from build123d import *

# Parameters (mm, degrees)
SKETCH_1_R                = 39.75
EXTRUDE_1_DEPTH           = 10
SKETCH_7_R                = 2.65
CUT_EXTRUDE_5_DEPTH       = 8
PATTERN_CIRCULAR_1_COUNT  = 2
PATTERN_CIRCULAR_1_ANGLE  = 25
F_1_THE_OTHER_WAY_COUNT   = 2
F_1_THE_OTHER_WAY_ANGLE   = 25
MIRROR_1_COPY_1_SKETCH_R  = 2.65
MIRROR_1_COPY_1_DEPTH     = 8
MIRROR_1_COPY_2_SKETCH_R  = 2.65
MIRROR_1_COPY_2_DEPTH     = 8
SKETCH_9_R                = 2.65
CUT_EXTRUDE_7_DEPTH       = 8
PATTERN_CIRCULAR_2_COUNT  = 2
CUT_EXTRUDE_START         = -10
CUT_EXTRUDE_8_DEPTH       = 10
CUT_EXTRUDE_13_DEPTH      = 4
SKETCH_12_R               = 25
EXTRUDE_2_DEPTH           = 10
SKETCH_16_R               = 21.4
CUT_EXTRUDE_14_DEPTH      = 6
CUT_EXTRUDE_10_DEPTH      = 58.09750448
CUT_EXTRUDE_10_DEPTH_BACK = 58.09750448
SKETCH_13_R               = 2.25
SKETCH_13_R_2             = 13.5
SKETCH_17_R               = 4.25
CUT_EXTRUDE_15_DEPTH      = 8
FILLET_1_R                = 2.5


# Read off the part's stored shape, not the designer's step: Вырез-Вытянуть8
with BuildPart() as part:
    # Эскиз1 → Бобышка-Вытянуть1 (new body)
    with BuildSketch(Plane.XY):
        Circle(SKETCH_1_R)
    extrude(amount=EXTRUDE_1_DEPTH)

    # Эскиз7 → Вырез-Вытянуть5 (cut)
    with BuildSketch(Plane(origin=(0, 39.75, 0), x_dir=(0, 0, -1), z_dir=(0, 1, 0))):
        with Locations(Location((-5, 0, 0), (0, 0, 90))):
            Circle(SKETCH_7_R)
    cut_extrude_5 = extrude(amount=-CUT_EXTRUDE_5_DEPTH, mode=Mode.SUBTRACT)

    # Круговой массив1: Вырез-Вытянуть5 ×2 about axis
    pattern_circular_1_axis = Axis((0, 0, 10), (0, 0, -1))
    for i in range(1, PATTERN_CIRCULAR_1_COUNT):
        add(cut_extrude_5.rotate(pattern_circular_1_axis, i * PATTERN_CIRCULAR_1_ANGLE / (PATTERN_CIRCULAR_1_COUNT - 1)), mode=Mode.SUBTRACT)

    # 1 the other way: Вырез-Вытянуть5 ×2 about axis
    f_1_the_other_way_axis = Axis((0, 0, 10), (0, 0, 1))
    for i in range(1, F_1_THE_OTHER_WAY_COUNT):
        add(cut_extrude_5.rotate(f_1_the_other_way_axis, i * F_1_THE_OTHER_WAY_ANGLE / (F_1_THE_OTHER_WAY_COUNT - 1)), mode=Mode.SUBTRACT)

    # Зеркальное отражение1: Вырез-Вытянуть5 across plane
    add(cut_extrude_5.mirror(Plane.ZX), mode=Mode.SUBTRACT)

    # Зеркальное отражение1 copy 1 sketch → Зеркальное отражение1 copy 1 (cut)
    with BuildSketch(Plane(origin=(16.799075904, -36.025734535, 0), x_dir=(0, 0, -1), z_dir=(0.4226182617407035, -0.906307787036648, 0))):
        with Locations((-5, 0)):
            Circle(MIRROR_1_COPY_1_SKETCH_R)
    extrude(amount=-MIRROR_1_COPY_1_DEPTH, mode=Mode.SUBTRACT)

    # Зеркальное отражение1 copy 2 sketch → Зеркальное отражение1 copy 2 (cut)
    with BuildSketch(Plane(origin=(-16.799075904, -36.025734535, 0), x_dir=(0, 0, -1), z_dir=(-0.42261826174069717, -0.9063077870366509, 0))):
        with Locations((-5, 0)):
            Circle(MIRROR_1_COPY_2_SKETCH_R)
    extrude(amount=-MIRROR_1_COPY_2_DEPTH, mode=Mode.SUBTRACT)

    # Эскиз9 → Вырез-Вытянуть7 (cut)
    with BuildSketch(Plane.ZY.offset(39.75)):
        with Locations((5, 0)):
            Circle(SKETCH_9_R)
    cut_extrude_7 = extrude(amount=-CUT_EXTRUDE_7_DEPTH, mode=Mode.SUBTRACT)

    # Круговой массив2: Вырез-Вытянуть7 ×2 about axis
    pattern_circular_2_axis = Axis((0, 0, 10), (0, 0, -1))
    for i in range(1, PATTERN_CIRCULAR_2_COUNT):
        add(cut_extrude_7.rotate(pattern_circular_2_axis, i * 360 / PATTERN_CIRCULAR_2_COUNT), mode=Mode.SUBTRACT)

    # Вырез-Вытянуть8 outline → Вырез-Вытянуть8 (cut)
    with BuildSketch(Plane(origin=(0, 0, 0), x_dir=(-1, 0, 0), z_dir=(0, 0, -1)).offset(CUT_EXTRUDE_START)):
        with BuildLine():
            Line((36.811173575, 15), (26.811173575, 15))
            Line((26.811173575, 15), (26.811173575, -15))
            Line((26.811173575, -15), (36.811173575, -15))
            ThreePointArc((36.811173575, -15), (39.75, 0), (36.811173575, 15))
        make_face()
    extrude(amount=CUT_EXTRUDE_8_DEPTH, mode=Mode.SUBTRACT)

    # Эскиз15 → Вырез-Вытянуть13 (cut)
    with BuildSketch(Plane.XY.offset(10)):
        Polygon((-1.767766953, 1.767766953), (1.767766953, -1.767766953), (33.587572106, 30.0520382), (30.0520382, 33.587572106), align=None)
    extrude(amount=-CUT_EXTRUDE_13_DEPTH, mode=Mode.SUBTRACT)

    # Эскиз12 → Бобышка-Вытянуть2 (add)
    with BuildSketch(Plane.XY):
        Circle(SKETCH_12_R)
    extrude(amount=-EXTRUDE_2_DEPTH)

    # Эскиз16 → Вырез-Вытянуть14 (cut)
    with BuildSketch(Plane(origin=(0, 0, -10), x_dir=(-1, 0, 0), z_dir=(0, 0, -1))):
        Circle(SKETCH_16_R)
    extrude(amount=-CUT_EXTRUDE_14_DEPTH, mode=Mode.SUBTRACT)

    # Эскиз13 → Вырез-Вытянуть10 (cut, two sides: drawn at the far end of the back side and taken through both)
    with BuildSketch(Plane.XY.offset(-CUT_EXTRUDE_10_DEPTH_BACK)):
        with Locations((17.5, 0)):
            Circle(SKETCH_13_R)
        with Locations((0, -17.5)):
            Circle(SKETCH_13_R)
        with Locations((-17.5, 0)):
            Circle(SKETCH_13_R)
        with Locations((0, 17.5)):
            Circle(SKETCH_13_R)
        Circle(SKETCH_13_R_2)
    extrude(amount=CUT_EXTRUDE_10_DEPTH + CUT_EXTRUDE_10_DEPTH_BACK, mode=Mode.SUBTRACT)

    # Эскиз17 → Вырез-Вытянуть15 (cut)
    with BuildSketch(Plane.XY.offset(10)):
        with Locations((0, 17.5)):
            Circle(SKETCH_17_R)
        with Locations((17.5, 0)):
            Circle(SKETCH_17_R)
        with Locations((0, -17.5)):
            Circle(SKETCH_17_R)
        with Locations((-17.5, 0)):
            Circle(SKETCH_17_R)
    extrude(amount=-CUT_EXTRUDE_15_DEPTH, mode=Mode.SUBTRACT)

    # Скругление1
    fillet_1_edges = [part.edges().sort_by_distance(p)[0] for p in [
        (20.48410737, 16.948573464, 6),
        (16.948573464, 20.48410737, 6),
        (-26.811173575, 15, 5),
        (-26.811173575, -15, 5),
    ]]
    fillet(fillet_1_edges, radius=FILLET_1_R - 0.0004)  # a hair under: the kernel refuses the full size
    fillet_1_2_edges = [part.edges().sort_by_distance(p)[0] for p in [
        (-36.811173575, -15, 5),
        (-36.811173575, 15, 5),
        (-1.259999544, -13.441071429, 6),
        (1.259999544, -13.441071429, 6),
        (13.441071429, -1.259999544, 6),
        (13.441071429, 1.259999544, 6),
        (-13.441071429, 1.259999544, 6),
        (-13.441071429, -1.259999544, 6),
        (-1.259999544, 13.441071429, 6),
        (1.259999544, 13.441071429, 6),
    ]]
    fillet(fillet_1_2_edges, radius=FILLET_1_R)


solid = part.part
Input: part model. Units: mm. Frame: model coordinates. A direction names the side the tool comes from. Give positions to 0.01 mm unless a question says otherwise; leave off trailing zeros. Order: outer loops, then holes, each group sorted by start corner. A loop starts at its lowest first (then second) coordinate and runs counter-clockwise, first axis right, second up. Notation, with made-up numbers: (78, 5) - (98, 5) arc R21 cw to (98, 43) - close; hole circle Ø5 at (-25, 7.25). An arc over 180 degrees is marked (long way). Answer as a JSON object with one key per item and string values. Group by question number.
Q1. Cut plane A-A, the plane z = -1.5. Output: boundary loops of the cut face in (x, y), then the cut area to 3 significant figures.
Q2. Cut plane B-B, the plane y = -17.5. Output: boundary loops of the cut face in (x, z), then the cut area to 3 significant figures.
Q3. Line query: probe 1 along Y at (x, z) = (0, -0.15); probe 2 along X at (y, z) = (0, 6.75); probe 3 along Y at (x, z) = (0, -8.6). Output: solid intervals per line, ascending.
Q4. First-contact query: pin 1 Ø5 at (y, z) = (8, -3.5) entering from -X; pin 2 Ø21.5 at (x, y) = (-1, 8) entering from -Z; pin 3 Ø4 at (x, z) = (29, 2) entering from -Y. Flat tips, straight axial feed; report the tip coordinate or a pass-through.
Q5. Cut plane C-C, the plane x = 0. Count the separate pieces of the cut face and the enclosed holes in it, then the cut area to 3 significant figures.
Q6. Cut plane D-D, the plane z = -8.25. Output: boundary loops of the cut face in (x, y), then the cut area to 3 significant figures.
Q7. Set-up query: faces 4 (the face through (-27.524, -14.248, 4.93)), 5 (the face through (13.45, 28.76, 5.04)), 6 (the face through (0, -31.75, 5)), 7 (the face through (35.806, -0.796, 7.528)), 8 (the face through (17.349, 19.877, 6.752)). Return all of +Z, -Z, +X, -X, +Y, -Y with unobstructed straight access to the full face (end or side cutting, diameter ignored); none if empty.
Q8. Mould query, pull axis Y, two halves, no side actions, for faces 1 (the face through (23.846, 7.509, -4.93)), 2 (the face through (0.57, 35.81, 2.41)), 3 (the face through (-27.563, 14.287, 4.93)). Classes: pulls with the +Y half, pulls with the -Y half, needs draft (parallel to the pull), parting line crosses it, or undercut.
Results:
{
 "1": {"outline": "circle Ø50 at (0, 0); hole circle Ø4.5 at (-17.5, 0); hole circle Ø27 at (0, 0); hole circle Ø4.5 at (0, -17.5); hole circle Ø4.5 at (0, 17.5); hole circle Ø4.5 at (17.5, 0)", "area": "1,330 mm^2"},
 "2": {"outline": "(-35.38, 0) - (-17.85, 0) - (-17.85, -10) - (-12.32, -10) - (-12.32, -4) - (-2.25, -4) - (-2.25, 2) - (-4.25, 2) - (-4.25, 10) - (-35.38, 10) - close; (2.25, -4) - (12.32, -4) - (12.32, -10) - (17.85, -10) - (17.85, 0) - (35.69, 0) - (35.69, 10) - (4.25, 10) - (4.25, 2) - (2.25, 2) - close", "area": "825 mm^2"},
 "3": {"probe 1": "-25 to -19.75, -15.25 to -13.5, 13.5 to 15.25, 19.75 to 25", "probe 2": "-26.81 to -21.75, 21.75 to 31.75", "probe 3": "-25 to -21.4, 21.4 to 25"},
 "4": {"pin 1": "x = -24.39", "pin 2": "z = -4", "pin 3": "y = -29.17"},
 "5": {"separate pieces": "4", "enclosed holes": "0", "area": "389 mm^2"},
 "6": {"outline": "circle Ø50 at (0, 0); hole circle Ø42.8 at (0, 0)", "area": "525 mm^2"},
 "7": {"face 4": "+Z, -Z, -X", "face 5": "none", "face 6": "-Y", "face 7": "+X", "face 8": "+Z"},
 "8": {"face 1": "parting line crosses it", "face 2": "needs draft", "face 3": "undercut"}
}
